The model under review builds one solid part; all positions refer to its coordinate system, in mm. Face numbers are marked on the shaded views. A direction names the side the tool comes from. Round coordinates to 2 decimals unless told otherwise and drop trailing zeros. Loops run counter-clockwise (first coordinate to the right, second up) from the corner with the lowest first, then second, coordinate; pieces in that order, holes last. Notation, with made-up numbers: M 80.25,18.25 L 139.25,18.25 A22 ccw 139.25,47.25 Z; hole C -17.5,-39.75 d8. An arc over 180 degrees is marked long. Answer as a JSON object with one key per item and string values. Group by question number.
Item 1: The part is to be moulded in two halves that separate along X. For the marked faces 1, 2 and 3, say which applies: +X half, -X half, draft (parallel to the pull), parting line (faces both ways), or undercut.
Item 2: To check wall thickness, follow line 1 (X direction, y = 6.5, z = 0); line 2 (Z direction, x = 0, y = 2.5); line 3 (X direction, y = 2.9, z = -7.5). State the ranges of each line that lie inside material, in increasing order.
Item 3: Consider section A-A (z = 12.5). Give the boundary of the cut face in (x, y).
Item 4: Insertion check: P1, Ø1.5, axis at x = 2.5, y = 19, coming from the -Z side; P2, Ø7, axis at x = 0, z = 12.5, coming from the +Y side; P3, Ø2, axis at x = 8.5, z = -3, coming from the +Y side. Each pin has a flat end and moves straight along its axis. Give the tip position at first contact, or say it passes through.
Item 5: Consider section C-C (x = 5.5). Give the boundary of the cut face in (y, z), and give its area (3 significant figures).
Item 6: Tool access review of the marked faces 4, 5 and 6: name each direction out of +Z, -Z, +X, -X, +Y, -Y from which nothing blocks a thin tool from reaching the whole face with its end or side.
Item 7: Consider section B-B (z = 2.5). Give the boundary of the cut face in (x, y), and give its area (3 significant figures).
Item 8: Consider section D-D (y = 19). Give the boundary of the cut face in (x, z).
```python
from build123d import *

# Parameters (mm, degrees)
SKETCH1_W           = 20
SKETCH1_H           = 40
BOSS_EXTRUDE1_DEPTH = 5
BOSS_EXTRUDE2_DEPTH = 20
SKETCH3_R           = 3
CUT_EXTRUDE1_DEPTH  = 15
LPATTERN1_COUNT     = 2
LPATTERN1_PITCH     = 20
SKETCH4_R           = 7.4
CUT_EXTRUDE2_DEPTH  = 15
SKETCH5_R           = 2
CUT_EXTRUDE3_DEPTH  = 50
CUT_EXTRUDE4_START  = -6
CUT_EXTRUDE4_DEPTH  = 40
CHAMFER1_SIZE       = 1
FILLET2_R           = 1
SKETCH7_W           = 2
SKETCH7_H           = 45.940909218
BOSS_EXTRUDE3_DEPTH = 5
LPATTERN2_COUNT     = 2
LPATTERN2_PITCH     = 18
FILLET3_R           = 1
CHAMFER2_SIZE       = 6
FILLET4_R           = 10


with BuildPart() as part:
    # Sketch1 → Boss-Extrude1 (new body)
    with BuildSketch(Plane(origin=(0, 0, 0), x_dir=(1, 0, 0), z_dir=(0, 1, 0))):
        Rectangle(SKETCH1_W, SKETCH1_H)
    extrude(amount=BOSS_EXTRUDE1_DEPTH)

    # Sketch2 → Boss-Extrude2 (add)
    with BuildSketch(Plane.ZY.offset(10)):
        Polygon((-5.650883497, 0), (-26.864086932, 21.213203436), (-48.077290368, 0), align=None)
    extrude(amount=-BOSS_EXTRUDE2_DEPTH)

    # Sketch3 → Cut-Extrude1 (cut)
    with BuildSketch(Plane(origin=(0, 5, 0), x_dir=(1, 0, 0), z_dir=(0, 1, 0))):
        with Locations((0, -12.5)):
            Circle(SKETCH3_R)
    cut_extrude1 = extrude(amount=-CUT_EXTRUDE1_DEPTH, mode=Mode.SUBTRACT)

    # LPattern1: Cut-Extrude1 ×2
    with Locations(*[(0, 0, -i * LPATTERN1_PITCH) for i in range(1, LPATTERN1_COUNT)]):
        add(cut_extrude1, mode=Mode.SUBTRACT)

    # Sketch4 → Cut-Extrude2 (cut)
    with BuildSketch(Plane(origin=(0, 5, 0), x_dir=(1, 0, 0), z_dir=(0, 1, 0))):
        with Locations((0, 7.5)):
            Circle(SKETCH4_R)
    extrude(amount=CUT_EXTRUDE2_DEPTH, mode=Mode.SUBTRACT)

    # Sketch5 → Cut-Extrude3 (cut)
    with BuildSketch(Plane(origin=(0, -2.825441748, -2.825441748), x_dir=(1, 0, 0), z_dir=(0, 0.707106781, 0.707106781))):
        with Locations((0, 26.49577804)):
            Circle(SKETCH5_R)
    extrude(amount=-CUT_EXTRUDE3_DEPTH, mode=Mode.SUBTRACT)

    # Sketch6 → Cut-Extrude4 (cut)
    with BuildSketch(Plane(origin=(0, -2.825441748, -2.825441748), x_dir=(1, 0, 0), z_dir=(0, 0.707106781, 0.707106781)).offset(CUT_EXTRUDE4_START)):
        Polygon((0, 30.24855479), (-3.25, 28.372166415), (-3.25, 24.619389665), (0, 22.743001291), (3.25, 24.619389665), (3.25, 28.372166415), align=None)
    extrude(amount=-CUT_EXTRUDE4_DEPTH, mode=Mode.SUBTRACT)

    # Chamfer1
    chamfer1_edges = [part.edges().sort_by_distance(p)[0] for p in [
        (-2, 15.909902577, -21.560786074),
    ]]
    chamfer(chamfer1_edges, length=CHAMFER1_SIZE)

    # Fillet2
    fillet2_edges = [part.edges().sort_by_distance(p)[0] for p in [
        (0, 0, -48.077290368),
        (-3, 0, 12.5),
        (-3, 0, -7.5),
        (0, 0, 20),
        (-10, 0, -14.038645184),
        (-1.625, 0, -41.451109482),
        (-3.25, 0, -37.47068865),
        (-1.625, 0, -33.490267818),
        (1.625, 0, -33.490267818),
        (3.25, 0, -37.47068865),
        (1.625, 0, -41.451109482),
        (10, 0, -14.038645184),
    ]]
    fillet(fillet2_edges, radius=FILLET2_R)

    # Sketch7 → Boss-Extrude3 (add)
    with BuildSketch(Plane(origin=(0, 5, 0), x_dir=(1, 0, 0), z_dir=(0, 1, 0))):
        with Locations((-9, 2.970454609)):
            Rectangle(SKETCH7_W, SKETCH7_H)
    boss_extrude3 = extrude(amount=BOSS_EXTRUDE3_DEPTH)

    # LPattern2: Boss-Extrude3 ×2
    with Locations(*[(i * LPATTERN2_PITCH, 0, 0) for i in range(1, LPATTERN2_COUNT)]):
        add(boss_extrude3)

    # Fillet3
    fillet3_edges = [part.edges().sort_by_distance(p)[0] for p in [
        (-8, 5, 4.674558252),
        (8, 5, 4.674558252),
    ]]
    fillet(fillet3_edges, radius=FILLET3_R)

    # Chamfer2
    chamfer2_edges = [part.edges().sort_by_distance(p)[0] for p in [
        (9, 10, 20),
    ]]
    chamfer(chamfer2_edges, length=CHAMFER2_SIZE)

    # Fillet4
    fillet4_edges = [part.edges().sort_by_distance(p)[0] for p in [
        (-9, 10, -15.650883497),
        (9, 10, -15.650883497),
    ]]
    fillet(fillet4_edges, radius=FILLET4_R)


solid = part.part
```
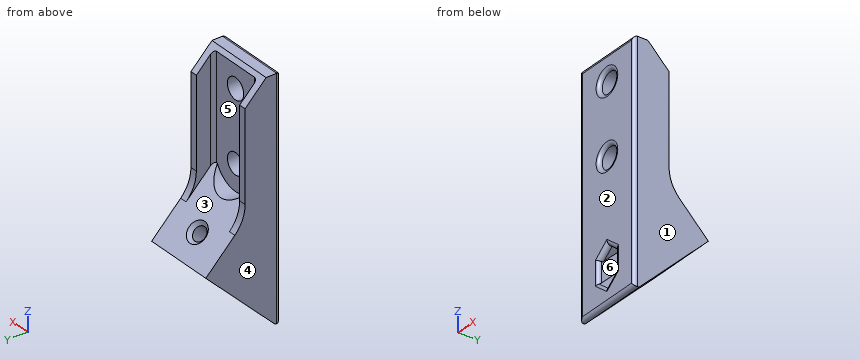
Geometry results:
{
 "1": {"face 1": "+X half", "face 2": "draft", "face 3": "undercut"},
 "2": {"line 1": "x = -10 to -8, 8 to 10", "line 2": "z = -45.58 to -40.28, -29.66 to -10.5, -4.5 to 9.5, 15.5 to 20", "line 3": "x = -10 to -3, 3 to 10"},
 "3": {"outline": "M -10,1 A1 ccw -9,0 L -4,0 A1 ccw -3,1 L -3,5 L -7,5 A1 cw -8,6 L -8,10 L -10,10 Z; M 3,1 A1 ccw 4,0 L 9,0 A1 ccw 10,1 L 10,10 L 8,10 L 8,6 A1 cw 7,5 L 3,5 Z"},
 "4": {"P1": "stops at z = -29.83", "P2": "stops at y = 5", "P3": "stops at y = 10"},
 "5": {"outline": "M 0,-45.66 A1 ccw 1.71,-46.37 L 21.21,-26.86 L 6.8,-12.45 L 5,-12.45 L 5,19 L 4,20 L 1,20 A1 ccw 0,19 Z", "area": "587 mm^2"},
 "6": {"face 4": "+Z, -Z, -X, +Y, -Y", "face 5": "+Z, +Y", "face 6": "none"},
 "7": {"outline": "M -10,1 A1 ccw -9,0 L 9,0 A1 ccw 10,1 L 10,10 L 8,10 L 8,6 A1 cw 7,5 L -7,5 A1 cw -8,6 L -8,10 L -10,10 Z", "area": "120 mm^2"},
 "8": {"outline": "M -10,-29.08 L 10,-29.08 L 10,-24.65 L -10,-24.65 Z"}
}
